from build123d import *

# Parameters (mm, degrees)
SKETCH1_R           = 1.5
BOSS_EXTRUDE3_DEPTH = 6


with BuildPart() as part:
    # Sketch1 → Boss-Extrude3 (new body)
    with BuildSketch(Plane.XY):
        with BuildLine():
            Line((20.05, 5), (0, 5))
            ThreePointArc((0, 5), (-5, 0), (0, -5))
            Line((0, -5), (22, -5))
            Line((22, -5), (26.72989842, 1.621129525))
            Line((26.72989842, 1.621129525), (77.820171744, 22.626880444))
            Line((77.820171744, 22.626880444), (84.10849538, 20.130806965))
            Line((84.10849538, 20.130806965), (85.272939558, 19.928397094))
            Line((85.272939558, 19.928397094), (85.958251837, 20.89133379))
            Line((85.958251837, 20.89133379), (87.122696015, 20.688923919))
            Line((87.122696015, 20.688923919), (87.808008293, 21.651860615))
            Line((87.808008293, 21.651860615), (88.972452471, 21.449450744))
            Line((88.972452471, 21.449450744), (89.657764749, 22.412387441))
            Line((89.657764749, 22.412387441), (90.822208927, 22.20997757))
            Line((90.822208927, 22.20997757), (91.507521206, 23.172914266))
            Line((91.507521206, 23.172914266), (92.671965384, 22.970504395))
            Line((92.671965384, 22.970504395), (93.357277662, 23.933441092))
            Line((93.357277662, 23.933441092), (91.646092305, 28.095393119))
            Line((91.646092305, 28.095393119), (84.329036858, 31.428307185))
            Line((84.329036858, 31.428307185), (20.05, 5))
        make_face()
        Circle(SKETCH1_R, mode=Mode.SUBTRACT)
        with Locations((22.020705275, 0.206842568)):
            Circle(SKETCH1_R, mode=Mode.SUBTRACT)
    extrude(amount=BOSS_EXTRUDE3_DEPTH)


solid = part.part
Build history of the part. All positions in model axes, mm. A direction names the side the tool comes from. Round coordinates to 2 decimals unless told otherwise and drop trailing zeros. Write each loop counter-clockwise with the first axis right and the second up, starting at its lowest first coordinate (ties: lowest second). Pieces come first, ordered by that corner, then holes. Notation, with made-up numbers: (-19.75, -32.75) -> (25.25, -32.75) arc R6 cw to (25.25, -26.75) -> close; hole circle Ø2 at (17, -21.5). An arc over 180 degrees is marked (long way). Write item = value, one per line.
(1) Band-saw the part on B-B (x = 18). Give the cut face in (y, z), then the cut area to 3 significant figures.
Answer:
outline = (-5, 0) -> (5, 0) -> (5, 6) -> (-5, 6) -> close
area = 60.0 mm2
(2) Band-saw the part on A-A (z = 3.1). Give the cut face in (x, y), then the cut area to 3 significant figures.
Answer:
outline = (0, -5) -> (22, -5) -> (26.73, 1.62) -> (77.82, 22.63) -> (84.11, 20.13) -> (85.27, 19.93) -> (85.96, 20.89) -> (87.12, 20.69) -> (87.81, 21.65) -> (88.97, 21.45) -> (89.66, 22.41) -> (90.82, 22.21) -> (91.51, 23.17) -> (92.67, 22.97) -> (93.36, 23.93) -> (91.65, 28.1) -> (84.33, 31.43) -> (20.05, 5) -> (0, 5) arc R5 ccw to start; hole circle Ø3 at (0, 0); hole circle Ø3 at (22.02, 0.21)
area = 722 mm2
(3) Two-plate mould, pull along X, no slides. Class faces 1 (the face through (-5, 0, 3)), 2 (the face through (80.92, 21.396, 2.958)), 3 (the face through (11, -5, 3)): pulls with the +X half, pulls with the -X half, needs draft (parallel to the pull), parting line crosses it, or undercut.
Answer:
face_1 = pulls with the -X half
face_2 = undercut
face_3 = needs draft
(4) Probe L1, parallel to Y at x = 8.5, z = 3.75; L2, parallel to X at y = 16.5, z = 3.9; L3, parallel to X at y = 25, z = 0.8. List the from-to ranges inside material, lowest first.
Answer:
L1 = -5 to 5
L2 = 48.02 to 62.92
L3 = 68.69 to 92.92
(5) Flat gauge pins, fed straight in: pin 1 (2.5 mm diameter, centred on x = 22.02, y = 0.21, fed in from +Z); pin 2 (1 mm diameter, centred on x = 52, z = 1, fed in from -Y); pin 3 (1.5 mm diameter, centred on x = 45, z = 1.5, fed in from +Y); pin 4 (1.5 mm diameter, centred on y = 7.5, z = 4.5, fed in from +X). Where does each tip first touch, or does it go through?
Answer:
pin_1 = through
pin_2 = 11.81
pin_3 = 15.57
pin_4 = 42.85
(6) Band-saw the part on C-C (y = -2.5). Give the cut face in (x, z).
Answer:
outline = (-4.33, 0) -> (23.79, 0) -> (23.79, 6) -> (-4.33, 6) -> close
(7) Tool access for faces 4 (the face through (10, 5, 3)), 5 (the face through (23.45, 0.66, 2.96)): list every direction of +Z, -Z, +X, -X, +Y, -Y with a clear straight run to the whole face (end or side of a thin tool).
Answer:
face_4 = +Z, -Z, -X, +Y
face_5 = +Z, -Z
